Verification items for the finished model (mm, model axes). Face numbers are marked on the shaded views. A direction names the side the tool comes from. Round coordinates to 2 decimals unless told otherwise and drop trailing zeros. Write each loop counter-clockwise with the first axis right and the second up, starting at its lowest first coordinate (ties: lowest second). Pieces come first, ordered by that corner, then holes. Notation, with made-up numbers: (72.5, 15.25) - (115.5, 15.25) arc R29 cw to (115.5, 51.25) - close; hole circle Ø3 at (38.25, 67.25). An arc over 180 degrees is marked (long way). Write each question's results on one line, items separated by ' | '.
```python
from build123d import *

# Parameters (mm, degrees)
BOSS_EXTRUDE1_DEPTH = 25
CUT_EXTRUDE1_REACH  = 33.464
SKETCH2_R           = 1.5
CUT_EXTRUDE2_REACH  = 34.094
SKETCH3_R           = 1.5
CUT_EXTRUDE3_REACH  = 32.033
SKETCH5_R           = 0.25
FILLET1_R           = 0.3
SKETCH6_R           = 3.05
CUT_EXTRUDE4_DEPTH  = 2
SKETCH7_R           = 3.05
CUT_EXTRUDE5_DEPTH  = 2
SKETCH9_R           = 4.5
BOSS_EXTRUDE2_DEPTH = 10.5
SKETCH10_R          = 0.75
CUT_EXTRUDE6_DEPTH  = 10.5
FILLET2_R           = 0.5


with BuildPart() as part:
    # Sketch1 → Boss-Extrude1 (new body)
    with BuildSketch(Plane.XY):
        Polygon((0, 0), (-14, 0), (-14, -4), (4, -4), (4, 9), (0, 9), align=None)
    extrude(amount=BOSS_EXTRUDE1_DEPTH)

    # Sketch2 → Cut-Extrude1 (cut, up to next)
    with BuildSketch(Plane.XZ.offset(4), mode=Mode.PRIVATE) as cut_extrude1_sk1:
        with Locations(Location((-9, 20, 0), (0, 0, 270))):
            Circle(SKETCH2_R)
    cut_extrude1_tool1 = extrude(cut_extrude1_sk1.sketch, amount=-CUT_EXTRUDE1_REACH, mode=Mode.PRIVATE) & part.part
    add(cut_extrude1_tool1.solids().sort_by_distance((-9, -4, 20))[0], mode=Mode.SUBTRACT)

    # Sketch3 → Cut-Extrude2 (cut, up to next)
    with BuildSketch(Plane(origin=(4, 0, 0), x_dir=(0, 0, -1), z_dir=(1, 0, 0)), mode=Mode.PRIVATE) as cut_extrude2_sk1:
        with Locations(Location((-5, 4.5, 0), (0, 0, 90))):
            Circle(SKETCH3_R)
    cut_extrude2_tool1 = extrude(cut_extrude2_sk1.sketch, amount=-CUT_EXTRUDE2_REACH, mode=Mode.PRIVATE) & part.part
    # Sketch3 → Cut-Extrude2 (cut, up to next)
    with BuildSketch(Plane(origin=(4, 0, 0), x_dir=(0, 0, -1), z_dir=(1, 0, 0)), mode=Mode.PRIVATE) as cut_extrude2_sk2:
        with Locations(Location((-20, 4.5, 0), (0, 0, 90))):
            Circle(SKETCH3_R)
    cut_extrude2_tool2 = extrude(cut_extrude2_sk2.sketch, amount=-CUT_EXTRUDE2_REACH, mode=Mode.PRIVATE) & part.part
    add(cut_extrude2_tool1.solids().sort_by_distance((4, 4.5, 5))[0], mode=Mode.SUBTRACT)
    add(cut_extrude2_tool2.solids().sort_by_distance((4, 4.5, 20))[0], mode=Mode.SUBTRACT)

    # Sketch5 → Cut-Extrude3 (cut, up to next)
    with BuildSketch(Plane.XY.offset(25), mode=Mode.PRIVATE) as cut_extrude3_sk1:
        Circle(SKETCH5_R)
    cut_extrude3_tool1 = extrude(cut_extrude3_sk1.sketch, amount=-CUT_EXTRUDE3_REACH, mode=Mode.PRIVATE) & part.part
    add(cut_extrude3_tool1.solids().sort_by_distance((0, 0, 25))[0], mode=Mode.SUBTRACT)

    # Fillet1
    fillet1_edges = [part.edges().sort_by_distance(p)[0] for p in [
        (0, 0.25, 12.5),
        (-0.25, 0, 12.5),
    ]]
    fillet(fillet1_edges, radius=FILLET1_R)

    # Sketch6 → Cut-Extrude4 (cut)
    with BuildSketch(Plane(origin=(4, 0, 0), x_dir=(0, 0, -1), z_dir=(1, 0, 0))):
        with Locations((-20, 4.5)):
            Circle(SKETCH6_R)
        with Locations((-5, 4.5)):
            Circle(SKETCH6_R)
    extrude(amount=-CUT_EXTRUDE4_DEPTH, mode=Mode.SUBTRACT)

    # Sketch7 → Cut-Extrude5 (cut)
    with BuildSketch(Plane.XZ.offset(4)):
        with Locations(Location((-9, 20, 0), (0, 0, 270))):
            Circle(SKETCH7_R)
    extrude(amount=-CUT_EXTRUDE5_DEPTH, mode=Mode.SUBTRACT)

    # Sketch9 → Boss-Extrude2 (add)
    with BuildSketch(Plane.XZ.offset(4)):
        with Locations(Location((-5, 7, 0), (0, 0, 90))):
            Circle(SKETCH9_R)
    extrude(amount=BOSS_EXTRUDE2_DEPTH)

    # Sketch10 → Cut-Extrude6 (cut)
    with BuildSketch(Plane.XZ.offset(14.5)):
        with Locations(Location((-5, 7, 0), (0, 0, 270))):
            Circle(SKETCH10_R)
    extrude(amount=-CUT_EXTRUDE6_DEPTH, mode=Mode.SUBTRACT)

    # Fillet2
    fillet2_edges = [part.edges().sort_by_distance(p)[0] for p in [
        (0, 9, 12.5),
        (4, 9, 12.5),
        (4, -4, 12.5),
        (-14, -4, 12.5),
        (-14, 0, 12.5),
    ]]
    fillet(fillet2_edges, radius=FILLET2_R)


solid = part.part
```
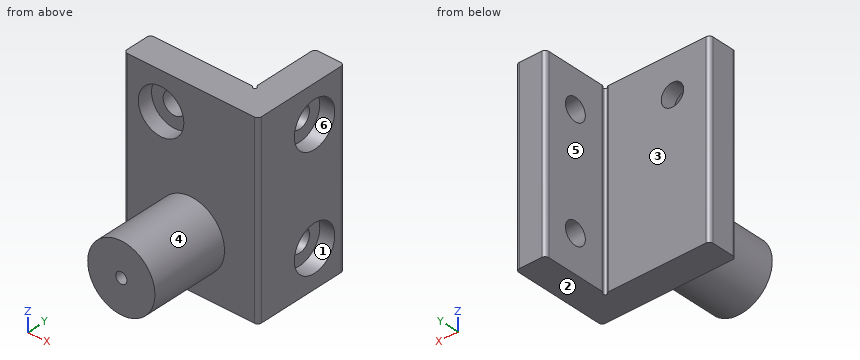
(1) Section check B-B (x = -10). Record the cut outline in (y, z).
Answer:
outline: (-4, 0) - (0, 0) - (0, 18.88) - (-2, 18.88) - (-2, 17.12) - (-4, 17.12) - close; (-4, 22.88) - (-2, 22.88) - (-2, 21.12) - (0, 21.12) - (0, 25) - (-4, 25) - close
(2) Section check A-A (y = 4.5). Record the cut outline in (x, z).
Answer:
outline: (0, 0) - (4, 0) - (4, 1.95) - (2, 1.95) - (2, 3.5) - (0, 3.5) - close; (0, 6.5) - (2, 6.5) - (2, 8.05) - (4, 8.05) - (4, 16.95) - (2, 16.95) - (2, 18.5) - (0, 18.5) - close; (0, 21.5) - (2, 21.5) - (2, 23.05) - (4, 23.05) - (4, 25) - (0, 25) - close
(3) Set-up check for the marked faces 4, 5 and 6: record each of +Z, -Z, +X, -X, +Y, -Y from which the full face is reachable in a straight line by a thin tool's end or side.
Answer:
face 4: -Y | face 5: +Z, -Z, -X, +Y | face 6: +X
(4) Thickness scan on L1, parallel to Z at x = 1.2, y = 4.5; L2, parallel to Y at x = 3, z = 5; L3, parallel to Y at x = 1.25, z = 9.5. Record the ranges inside material, lowest first.
Answer:
L1: 0 to 3.5, 6.5 to 18.5, 21.5 to 25 | L2: -4 to 1.45, 7.55 to 9 | L3: -4 to 9
(5) Mould release check, pull along Z, two halves, no side actions. Record for the marked faces 1, 2 and 3: released by +Z, released by -Z, zero draft, split by the parting line, or undercut.
Answer:
face 1: undercut | face 2: released by -Z | face 3: zero draft
(6) Section check D-D (y = -3). Record the cut outline in (x, z), plus the area to 3 significant figures.
Answer:
outline: (-14, 0) - (4, 0) - (4, 25) - (-14, 25) - close; hole circle Ø6.1 at (-9, 20) | area: 421 mm2
(7) Go/stop test with flat-tipped pins: pin 1 Ø5 at (x, z) = (-10.5, 21.5) entering from -Y; pin 2 Ø5 at (x, z) = (-9, 20) entering from -Y; pin 3 Ø7 at (y, z) = (4.5, 20) entering from -X. Record where each tip stops, or that it passes through.
Answer:
pin 1: y = -4 | pin 2: y = -2 | pin 3: x = 0
(8) Section check C-C (z = 16.25). Record the cut outline in (x, y).
Answer:
outline: (-14, -3.5) arc R0.5 ccw to (-13.5, -4) - (3.5, -4) arc R0.5 ccw to (4, -3.5) - (4, 8.5) arc R0.5 ccw to (3.5, 9) - (0.5, 9) arc R0.5 ccw to (0, 8.5) - (0, 0.46) arc R0.3 ccw to (0.14, 0.21) arc R0.25 cw (long way) to (-0.21, -0.14) arc R0.3 ccw to (-0.46, 0) - (-13.5, 0) arc R0.5 ccw to (-14, -0.5) - close
